Source: CAD feature listing. Evaluate the final solid. Frame: model axes, mm. Face numbers are marked on the shaded views. A direction names the side the tool comes from. Round coordinates to 2 decimals unless told otherwise and drop trailing zeros. Loops run counter-clockwise (first coordinate to the right, second up) from the corner with the lowest first, then second, coordinate; pieces in that order, holes last. Notation, with made-up numbers: M 8,23.5 L 35,23.5 A14 cw 35,39.5 Z; hole C 20.25,8.25 d2. An arc over 180 degrees is marked long. Answer as a JSON object with one key per item and string values.
from build123d import *

# Parameters (mm, degrees)
F0_W     = 70.33
F0_H     = 70.33
F1_DEPTH = 20
F2_T     = -0.3
F0_H_2   = 32
F3_DEPTH = 20
F4_T     = -0.3


# Not quite as in the source:
# - a shell that OpenCascade refuses in one call is made with other operations: the cavity is built on its own and cut out


with BuildPart() as f1:
    # F0 (on Front) → F1 (new body)
    with BuildSketch(Plane.XZ):
        Rectangle(F0_W, F0_H)
    extrude(amount=F1_DEPTH)

    # F2
    f2_openings = [f1.faces().sort_by_distance(p)[0] for p in [
        (0, -20, 0),
    ]]
    offset(amount=F2_T, openings=f2_openings)

    # F0 (on Front) → F3 (join)
    with BuildSketch(Plane.XZ):
        with Locations((0, 51.165)):
            Rectangle(F0_W, F0_H_2)
    extrude(amount=F3_DEPTH)

    # F4: a shell. OpenCascade refuses it in one call, so the cavity is built on its own and cut out:
    # the body offset inwards by the wall thickness, plus a prism from it out through each open face.
    f4_core = offset(f1.part, amount=F4_T, kind=Kind.INTERSECTION, mode=Mode.PRIVATE)
    f4_exits = [f4_core.faces().sort_by_distance(p)[0] for p in [
        (0, -19.7, 51.015),
    ]]
    add(f4_core, mode=Mode.SUBTRACT)
    extrude(f4_exits, amount=-F4_T, mode=Mode.SUBTRACT)


solid = f1.part
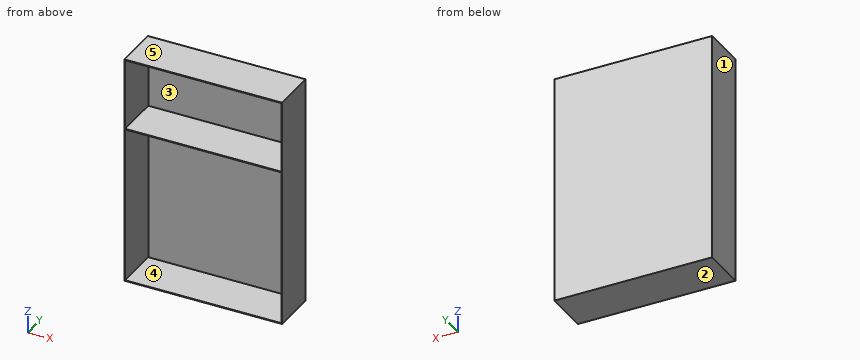
Item 1: Section B-B on z = -7.5. Return the cut outline in (x, y) (3 decimals), then the cut area to 3 significant figures.
Answer sheet:
{"outline": "M -35.165,-20 L -34.865,-20 L -34.865,-0.3 L 34.865,-0.3 L 34.865,-20 L 35.165,-20 L 35.165,0 L -35.165,0 Z", "area": "32.9 mm²"}
Item 2: Line query: probe 1 along Z at (x, y) = (9.5, -3.5) (3 decimals); probe 2 along X at (y, z) = (-11.5, -6) (3 decimals); probe 3 along Y at (x, z) = (-18, 20.5). Output: solid intervals per line, ascending. Write a range as from..to.
Answer sheet:
{"probe 1": "z = -35.165..-34.865, 34.865..35.165, 66.865..67.165", "probe 2": "x = -35.165..-34.865, 34.865..35.165", "probe 3": "y = -0.3..0"}
Item 3: Pull-direction query (X, two-part tool) for the marked faces 1, 2 and 3; classes: pulls with the +X half, pulls with the -X half, needs draft (parallel to the pull), parting line crosses it, or undercut.
Answer sheet:
{"face 1": "pulls with the -X half", "face 2": "needs draft", "face 3": "undercut"}
Item 4: Section C-C on x = 30. Return the cut outline in (y, z) (3 decimals), then the cut area to 3 significant figures.
Answer sheet:
{"outline": "M -20,-35.165 L 0,-35.165 L 0,67.165 L -20,67.165 L -20,66.865 L -0.3,66.865 L -0.3,35.165 L -20,35.165 L -20,34.865 L -0.3,34.865 L -0.3,-34.865 L -20,-34.865 Z", "area": "48.4 mm²"}
Item 5: Section A-A on y = -15.75. Return the cut outline in (x, z) (3 decimals).
Answer sheet:
{"outline": "M -35.165,-35.165 L 35.165,-35.165 L 35.165,67.165 L -35.165,67.165 Z; hole M -34.865,-34.865 L 34.865,-34.865 L 34.865,34.865 L -34.865,34.865 Z; hole M -34.865,35.165 L 34.865,35.165 L 34.865,66.865 L -34.865,66.865 Z"}
Item 6: Access query for the marked faces 4 and 5. Directions: +Z, -Z, +X, -X, +Y, -Y. A direction counts if a zero-diameter tool reaches every point of the face in a straight line with its end or side. Return the directions, or none.
Answer sheet:
{"face 4": "-Y", "face 5": "+Z, +X, -X, +Y, -Y"}
Item 7: Contact query for a flat-ended pin moving along its axis: pin 1 Ø3 at (x, z) = (21.5, 30.5) entering from -Y. Output: stop coordinate, or through.
Answer sheet:
{"pin 1": "stops at y = -0.3"}
